Check sheet for the modelled part. Datum: model origin and axes. Units: mm. A direction names the side the tool comes from. Give positions to 0.01 mm unless a question says otherwise; leave off trailing zeros. Order: outer loops, then holes, each group sorted by start corner. A loop starts at its lowest first (then second) coordinate and runs counter-clockwise, first axis right, second up.
```python
from build123d import *

# Parameters (mm, degrees)
CROQUIS1_W                   = 100
CROQUIS1_H                   = 60
CROQUIS1_R                   = 1.5
SALIENTE_EXTRUIR1_DEPTH      = 10
SALIENTE_EXTRUIR2_DEPTH      = 2
SALIENTE_EXTRUIR2_DEPTH_BACK = 3
CROQUIS1_2_W                 = 92
CROQUIS1_2_H                 = 46
CROQUIS2_W                   = 12
CROQUIS2_H                   = 14
CROQUIS2_W_2                 = 14
CORTAR_EXTRUIR1_DEPTH        = 5
CORTAR_EXTRUIR2_START        = -5
CROQUIS3_W                   = 12
CROQUIS3_H                   = 46
CORTAR_EXTRUIR2_DEPTH        = 5
MATRIZL1_COUNT               = 2
MATRIZL1_PITCH               = 80
CROQUIS4_W                   = 7
CROQUIS4_H                   = 7
CORTAR_EXTRUIR3_DEPTH        = 100
MATRIZL2_COUNT               = 2
MATRIZL2_PITCH               = 96


with BuildPart() as part:
    # Croquis1 → Saliente-Extruir1 (new body)
    with BuildSketch(Plane(origin=(0, 0, 0), x_dir=(1, 0, 0), z_dir=(0, 1, 0))):
        Rectangle(CROQUIS1_W, CROQUIS1_H)
        Polygon((-46, 20), (-25, 20), (-25, 24), (25, 24), (25, 20), (46, 20), (46, -26), (-46, -26), align=None, mode=Mode.SUBTRACT)
        with Locations(Location((-38, 25, 0), (0, 0, 270))):
            Circle(CROQUIS1_R, mode=Mode.SUBTRACT)
        with Locations(Location((-28, 25, 0), (0, 0, 270))):
            Circle(CROQUIS1_R, mode=Mode.SUBTRACT)
        with Locations(Location((28, 25, 0), (0, 0, 270))):
            Circle(CROQUIS1_R, mode=Mode.SUBTRACT)
        with Locations(Location((38, 25, 0), (0, 0, 270))):
            Circle(CROQUIS1_R, mode=Mode.SUBTRACT)
    extrude(amount=SALIENTE_EXTRUIR1_DEPTH)

    # Croquis1<2> → Saliente-Extruir2 (add, two sides: drawn at the far end of the back side and taken through both)
    with BuildSketch(Plane(origin=(0, 0, 0), x_dir=(1, 0, 0), z_dir=(0, 1, 0)).offset(-SALIENTE_EXTRUIR2_DEPTH_BACK)):
        with Locations((0, -3)):
            Rectangle(CROQUIS1_2_W, CROQUIS1_2_H)
    extrude(amount=SALIENTE_EXTRUIR2_DEPTH + SALIENTE_EXTRUIR2_DEPTH_BACK)

    # Croquis2 → Cortar-Extruir1 (cut)
    with BuildSketch(Plane(origin=(0, 2, 0), x_dir=(1, 0, 0), z_dir=(0, 1, 0))):
        with Locations((-22, -1)):
            Rectangle(CROQUIS2_W, CROQUIS2_H)
        with Locations((24, -1)):
            Rectangle(CROQUIS2_W_2, CROQUIS2_H)
    extrude(amount=-CORTAR_EXTRUIR1_DEPTH, mode=Mode.SUBTRACT)

    # Croquis3 → Cortar-Extruir2 (cut)
    with BuildSketch(Plane(origin=(0, 2, 0), x_dir=(1, 0, 0), z_dir=(0, 1, 0)).offset(CORTAR_EXTRUIR2_START)):
        with Locations((40, -3)):
            Rectangle(CROQUIS3_W, CROQUIS3_H)
    cortar_extruir2 = extrude(amount=CORTAR_EXTRUIR2_DEPTH, mode=Mode.SUBTRACT)

    # MatrizL1: Cortar-Extruir2 ×2
    with Locations(*[(-i * MATRIZL1_PITCH, 0, 0) for i in range(1, MATRIZL1_COUNT)]):
        add(cortar_extruir2, mode=Mode.SUBTRACT)

    # Croquis4 → Cortar-Extruir3 (cut)
    with BuildSketch(Plane.ZY.offset(-46)):
        with Locations((0, 5)):
            Rectangle(CROQUIS4_W, CROQUIS4_H)
    cortar_extruir3 = extrude(amount=-CORTAR_EXTRUIR3_DEPTH, mode=Mode.SUBTRACT)

    # MatrizL2: Cortar-Extruir3 ×2
    with Locations(*[(-i * MATRIZL2_PITCH, 0, 0) for i in range(1, MATRIZL2_COUNT)]):
        add(cortar_extruir3, mode=Mode.SUBTRACT)


solid = part.part
```
(1) Gauge pin test, flat ends, axial feed: pin 1 Ø1.5 at (y, z) = (-1.5, 8.5) entering from -X; pin 2 Ø11 at (x, z) = (-10.5, 14.5) entering from +Y; pin 3 Ø1.5 at (x, z) = (33, -1.5) entering from +Y; pin 4 Ø12 at (x, z) = (31.5, 23) entering from +Y. Record the tip position at first contact, or that the pin passes through.
Response values:
pin 1: stops at x = -34
pin 2: stops at y = 2
pin 3: stops at y = 1.5
pin 4: stops at y = 10
(2) Cross-section at C-C on y = 6.5. Enter the section's corners in (x, z), then the cut area to 3 significant figures.
Response values:
outline: (-50, -30) - (50, -30) - (50, -3.5) - (46, -3.5) - (46, -20) - (25, -20) - (25, -24) - (-25, -24) - (-25, -20) - (-46, -20) - (-46, -3.5) - (-50, -3.5) - close; (-50, 3.5) - (-46, 3.5) - (-46, 26) - (46, 26) - (46, 3.5) - (50, 3.5) - (50, 30) - (-50, 30) - close; hole circle Ø3 at (-38, -25); hole circle Ø3 at (-28, -25); hole circle Ø3 at (28, -25); hole circle Ø3 at (38, -25)
area: 1,480 mm2
(3) Material ranges on L1, parallel to X at y = 3.5, z = -25; L2, parallel to X at y = -0.75, z = -0.5; L3, parallel to Z at x = 40, y = 7.25, recorded low to high.
Response values:
L1: x = -50 to -39.5, -36.5 to -29.5, -26.5 to 26.5, 29.5 to 36.5, 39.5 to 50
L2: x = -34 to -28, -16 to 17, 31 to 34
L3: z = -30 to -20, 26 to 30
(4) Cross-section at B-B on x = 41. Enter the section's corners in (y, z), then the cut area to 3 significant figures.
Response values:
outline: (0, -30) - (10, -30) - (10, -20) - (0, -20) - close; (0, 26) - (10, 26) - (10, 30) - (0, 30) - close
area: 140 mm2
(5) Cross-section at D-D on x = -38. Enter the section's corners in (y, z), then the cut area to 3 significant figures.
Response values:
outline: (0, -30) - (10, -30) - (10, -26.5) - (0, -26.5) - close; (0, -23.5) - (10, -23.5) - (10, -20) - (0, -20) - close; (0, 26) - (10, 26) - (10, 30) - (0, 30) - close
area: 110 mm2
(6) Set-up check for faces 4 (the face through (-48, 5, 3.5)), 5 (the face through (17, 0, 1)), 6 (the face through (0, 2, 15)), 7 (the face through (-31, 1.5, 0)): record each of +Z, -Z, +X, -X, +Y, -Y from which the full face is reachable in a straight line by a thin tool's end or side.
Response values:
face 4: +X, -X
face 5: +Y, -Y
face 6: +Y
face 7: +X, -X, +Y
(7) Release check for a two-part mould opening along X. For faces 1 (the face through (50, 0.5, 0.4)), 2 (the face through (-1, 5, 30)), 3 (the face through (-16, 0, 1)) record: released by +X, released by -X, zero draft, split by the parting line, or undercut.
Response values:
face 1: released by +X
face 2: zero draft
face 3: undercut
(8) Cross-section at A-A on z = -25. Enter the section's corners in (x, y), then the cut area to 3 significant figures.
Response values:
outline: (-50, 0) - (-39.5, 0) - (-39.5, 10) - (-50, 10) - close; (-36.5, 0) - (-29.5, 0) - (-29.5, 10) - (-36.5, 10) - close; (-26.5, 0) - (26.5, 0) - (26.5, 10) - (-26.5, 10) - close; (29.5, 0) - (36.5, 0) - (36.5, 10) - (29.5, 10) - close; (39.5, 0) - (50, 0) - (50, 10) - (39.5, 10) - close
area: 880 mm2
